from build123d import *

# Parameters (mm, degrees)
BOSS_EXTRUDE1_DEPTH = 7.9
SKETCH2_W           = 25
SKETCH2_H           = 13.1
SKETCH2_R           = 1.349845
BOSS_EXTRUDE2_DEPTH = 7.75
SKETCH2_4_R         = 2.499995
SKETCH2_4_R_2       = 1.349845
CUT_EXTRUDE1_DEPTH  = 23.498
SKETCH2_6_R         = 2.6999438
SKETCH2_6_R_2       = 1.349845
CUT_EXTRUDE2_DEPTH  = 2.5


with BuildPart() as part:
    # Sketch1 → Boss-Extrude1 (new body)
    with BuildSketch(Plane.XY):
        with BuildLine():
            Line((-5, 10.5), (-12.5, 10.5))
            Line((-12.5, 10.5), (-12.5, -10.5))
            Line((-12.5, -10.5), (12.5, -10.5))
            Line((12.5, -10.5), (12.5, 10.5))
            Line((12.5, 10.5), (5, 10.5))
            ThreePointArc((5, 10.5), (0, 15.5), (-5, 10.5))
        make_face()
    extrude(amount=BOSS_EXTRUDE1_DEPTH)

    # Sketch2 → Boss-Extrude2 (add)
    with BuildSketch(Plane(origin=(0, -2.24999999, 0), x_dir=(1, 0, 0), z_dir=(0, 1, 0))):
        with Locations((0, -14.45)):
            Rectangle(SKETCH2_W, SKETCH2_H)
        with Locations((6.00015, -14.45)):
            Circle(SKETCH2_R, mode=Mode.SUBTRACT)
    extrude(amount=BOSS_EXTRUDE2_DEPTH)

    # Sketch2<4> → Cut-Extrude1 (cut)
    with BuildSketch(Plane(origin=(0, -2.24999999, 0), x_dir=(1, 0, 0), z_dir=(0, 1, 0))):
        with Locations((0, -14.45)):
            Circle(SKETCH2_4_R)
        with Locations((-6.00015, -14.45)):
            Circle(SKETCH2_4_R_2)
    extrude(amount=CUT_EXTRUDE1_DEPTH, mode=Mode.SUBTRACT)

    # Sketch2<6> → Cut-Extrude2 (cut)
    with BuildSketch(Plane(origin=(0, -2.24999999, 0), x_dir=(1, 0, 0), z_dir=(0, 1, 0))):
        with Locations((6.00015, -14.45)):
            Circle(SKETCH2_6_R)
        with Locations((6.00015, -14.45)):
            Circle(SKETCH2_6_R_2, mode=Mode.SUBTRACT)
        with Locations((-6.00015, -14.45)):
            Circle(SKETCH2_6_R)
        with Locations((-6.00015, -14.45)):
            Circle(SKETCH2_6_R_2, mode=Mode.SUBTRACT)
    extrude(amount=CUT_EXTRUDE2_DEPTH, mode=Mode.SUBTRACT)


solid = part.part
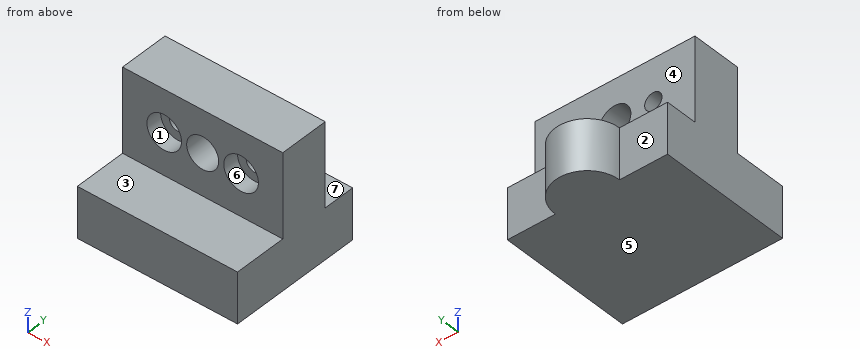
CAD build for the part. Positions are in the model's coordinates, mm. Face numbers are marked on the shaded views. A direction names the side the tool comes from. Coordinates: 2 decimals unless noted, no trailing zeros. Write each loop counter-clockwise with the first axis right and the second up, starting at its lowest first coordinate (ties: lowest second). Pieces come first, ordered by that corner, then holes. Notation, with made-up numbers: M -21,11 L 31,11 A17 ccw 31,30 Z; hole C 4,-20 d5. An arc over 180 degrees is marked long. Return JSON: item names as keys, results as strings.
Item 1: Probe line 1 (X direction, y = -0.6, z = 14.45); line 2 (X direction, y = 4.1, z = 14.45); line 3 (Z direction, x = 0, y = 0.75). List the from-to ranges inside material, lowest first. Write a range as from..to.
Findings below:
{"line 1": "x = -12.5..-8.7, -3.3..-2.5, 2.5..3.3, 8.7..12.5", "line 2": "x = -12.5..-7.35, -4.65..-2.5, 2.5..4.65, 7.35..12.5", "line 3": "z = 0..11.95, 16.95..21"}
Item 2: Which spindle directions (+Z, -Z, +X, -X, +Y, -Y) get a long thin tool onto all of the face, cutting with end or side? Do the marked faces 1, 2, 3 and 4. Say none if no direction does.
Findings below:
{"face 1": "-Y", "face 2": "+Z, -Z, -X, +Y", "face 3": "+Z, +X, -X, -Y", "face 4": "+Z, +X, -X, +Y"}
Item 3: Slice it at C-C, the plane y = -1.5. Write the cut outline in (x, z).
Findings below:
{"outline": "M -12.5,0 L 12.5,0 L 12.5,21 L -12.5,21 Z; hole C -6,14.45 d5.4; hole C 0,14.45 d5; hole C 6,14.45 d5.4"}
Item 4: Drop flat-ended pins along their axis: pin 1 Ø2.5 at (x, y) = (0.5, -7.5) entering from +Z; pin 2 Ø1.6 at (x, z) = (6, 13) entering from -Y; pin 3 Ø4 at (x, y) = (-0.5, 10) entering from -Z; pin 4 Ø5 at (x, z) = (8, 18) entering from +Y. Give the stop position or say it passes through.
Findings below:
{"pin 1": "stops at z = 7.9", "pin 2": "stops at y = 0.25", "pin 3": "stops at z = 0", "pin 4": "stops at y = 5.5"}
Item 5: Slice it at D-D, the plane x = 10.25. Write the cut outline in (y, z).
Findings below:
{"outline": "M -10.5,0 L 10.5,0 L 10.5,7.9 L 5.5,7.9 L 5.5,21 L -2.25,21 L -2.25,7.9 L -10.5,7.9 Z"}
Item 6: Slice it at B-B, the plane x = 0. Write the cut outline in (y, z).
Findings below:
{"outline": "M -10.5,0 L 15.5,0 L 15.5,7.9 L 5.5,7.9 L 5.5,11.95 L -2.25,11.95 L -2.25,7.9 L -10.5,7.9 Z; M -2.25,16.95 L 5.5,16.95 L 5.5,21 L -2.25,21 Z"}
Item 7: Two-plate mould, pull along Z, no slides. Class the marked faces 5, 6 and 7: +Z half, -Z half, draft (parallel to the pull), parting line (faces both ways), or undercut.
Findings below:
{"face 5": "-Z half", "face 6": "undercut", "face 7": "+Z half"}
Item 8: Slice it at A-A, the plane z = 14.45. Write the cut outline in (x, y).
Findings below:
{"outline": "M -12.5,-2.25 L -8.7,-2.25 L -8.7,0.25 L -7.35,0.25 L -7.35,5.5 L -12.5,5.5 Z; M -4.65,0.25 L -3.3,0.25 L -3.3,-2.25 L -2.5,-2.25 L -2.5,5.5 L -4.65,5.5 Z; M 2.5,-2.25 L 3.3,-2.25 L 3.3,0.25 L 4.65,0.25 L 4.65,5.5 L 2.5,5.5 Z; M 7.35,0.25 L 8.7,0.25 L 8.7,-2.25 L 12.5,-2.25 L 12.5,5.5 L 7.35,5.5 Z"}
